CAD build for the part. Positions are in the model's coordinates, mm. Coordinates: 2 decimals unless noted, no trailing zeros. Loops run counter-clockwise (first coordinate to the right, second up) from the corner with the lowest first, then second, coordinate; pieces in that order, holes last. Notation, with made-up numbers: (74, -12.75) -> (122, -12.75) arc R20 ccw to (122, 9.25) -> close; hole circle Ø10 at (9, -33.75). An arc over 180 degrees is marked (long way). Write each question's results on one line, items separated by ' | '.
```python
from build123d import *

# Parameters (mm, degrees)
CROQUIS1_W              = 108
CROQUIS1_H              = 71
SALIENTE_EXTRUIR1_DEPTH = 1.5
CROQUIS2_W              = 8
CROQUIS2_H              = 3
CROQUIS2_W_2            = 12
CORTAR_EXTRUIR1_DEPTH   = 3
CROQUIS4_W              = 8
CROQUIS4_H              = 3
SALIENTE_EXTRUIR2_DEPTH = 3
REDONDEO1_R             = 4
CROQUIS5_R              = 1.5
CORTAR_EXTRUIR2_DEPTH   = 13
SIMETR_A2_START         = -1.5
SIMETR_A2_OUTLINE_R     = 1.5
SIMETR_A2_DEPTH         = 3
SIMETR_A2_2_DEPTH       = 3
CROQUIS6_W              = 3
CROQUIS6_H              = 14
CROQUIS6_H_2            = 8
CORTAR_EXTRUIR3_DEPTH   = 3
CROQUIS7_W              = 3.217414859
CROQUIS7_H              = 7.6
CORTAR_EXTRUIR4_DEPTH   = 73
CROQUIS10_W             = 12.8
CROQUIS10_H             = 9.989091156
CORTAR_EXTRUIR7_DEPTH   = 10
CROQUIS11_W             = 12.481361742
CROQUIS11_H             = 10
CORTAR_EXTRUIR8_DEPTH   = 10
CROQUIS12_R             = 2
CROQUIS12_R_2           = 3.661926667
CROQUIS12_R_3           = 5
CROQUIS12_W             = 4.5
CROQUIS12_H             = 7
CORTAR_EXTRUIR9_DEPTH   = 10
CORTAR_EXTRUIR10_DEPTH  = 10


# Read off the part's stored shape, not the designer's step: Simetría2
with BuildPart() as part:
    # Croquis1 → Saliente-Extruir1 (new, symmetric)
    with BuildSketch(Plane(origin=(0, 0, 0), x_dir=(0, 0, -1), z_dir=(1, 0, 0))):
        Rectangle(CROQUIS1_W, CROQUIS1_H)
    extrude(amount=SALIENTE_EXTRUIR1_DEPTH, both=True)

    # Croquis2 → Cortar-Extruir1 (cut)
    with BuildSketch(Plane.ZY.offset(1.5)):
        with Locations((-8, -34)):
            Rectangle(CROQUIS2_W, CROQUIS2_H)
        with Locations((8, -34)):
            Rectangle(CROQUIS2_W, CROQUIS2_H)
        with Locations((48, 34)):
            Rectangle(CROQUIS2_W_2, CROQUIS2_H)
        with Locations((24, 34)):
            Rectangle(CROQUIS2_W, CROQUIS2_H)
        with Locations((8, 34)):
            Rectangle(CROQUIS2_W, CROQUIS2_H)
        with Locations((-8, 34)):
            Rectangle(CROQUIS2_W, CROQUIS2_H)
        with Locations((-24, 34)):
            Rectangle(CROQUIS2_W, CROQUIS2_H)
        with Locations((-48, 34)):
            Rectangle(CROQUIS2_W_2, CROQUIS2_H)
    extrude(amount=-CORTAR_EXTRUIR1_DEPTH, mode=Mode.SUBTRACT)

    # Croquis4 → Saliente-Extruir2 (add)
    with BuildSketch(Plane.ZY.offset(1.5)):
        with Locations((16, 37)):
            Rectangle(CROQUIS4_W, CROQUIS4_H)
    extrude(amount=-SALIENTE_EXTRUIR2_DEPTH)

    # Redondeo1
    redondeo1_edges = [part.edges().sort_by_distance(p)[0] for p in [
        (0, 38.5, 20),
        (0, 38.5, 12),
    ]]
    fillet(redondeo1_edges, radius=REDONDEO1_R - 0.0001)  # a hair under: the kernel refuses the full size

    # Croquis5 → Cortar-Extruir2 (cut)
    with BuildSketch(Plane.ZY.offset(1.5)):
        with Locations((16, 33.5)):
            Circle(CROQUIS5_R)
    extrude(amount=-CORTAR_EXTRUIR2_DEPTH, mode=Mode.SUBTRACT)

    # Simetría2 outline → Simetría2 (cut)
    with BuildSketch(Plane.YZ.offset(SIMETR_A2_START)):
        with BuildLine():
            ThreePointArc((-34.5, 12), (-35.00401717, 12.031881215), (-35.5, 12.127016654))
            Line((-35.5, 12.127016654), (-35.5, 12))
            Line((-35.5, 12), (-34.5, 12))
        make_face()
        with Locations((-33.5, 16)):
            Circle(SIMETR_A2_OUTLINE_R)
    extrude(amount=SIMETR_A2_DEPTH, mode=Mode.SUBTRACT)

    # Simetr_a2 2 outline → Simetr_a2 2 (add)
    with BuildSketch(Plane.YZ.offset(SIMETR_A2_START)):
        with BuildLine():
            ThreePointArc((-35.5, 20), (-37.66227766, 18.576506397), (-38.5, 16.127016654))
            Line((-38.5, 16.127016654), (-38.5, 16))
            ThreePointArc((-38.5, 16), (-37.66227766, 13.550510257), (-35.5, 12.127016654))
            Line((-35.5, 12.127016654), (-35.5, 20))
        make_face()
    extrude(amount=SIMETR_A2_2_DEPTH)

    # Croquis6 → Cortar-Extruir3 (cut)
    with BuildSketch(Plane.ZY.offset(1.5)):
        with Locations((52.5, -28.5)):
            Rectangle(CROQUIS6_W, CROQUIS6_H)
        with Locations((52.5, -6.5)):
            Rectangle(CROQUIS6_W, CROQUIS6_H_2)
        with Locations((52.5, 6.5)):
            Rectangle(CROQUIS6_W, CROQUIS6_H_2)
        with Locations((52.5, 28.5)):
            Rectangle(CROQUIS6_W, CROQUIS6_H)
    extrude(amount=-CORTAR_EXTRUIR3_DEPTH, mode=Mode.SUBTRACT)

    # Croquis7 → Cortar-Extruir4 (cut)
    with BuildSketch(Plane(origin=(0, 32.5, 0), x_dir=(1, 0, 0), z_dir=(0, 1, 0))):
        with Locations((-0.10870743, 50.2)):
            Rectangle(CROQUIS7_W, CROQUIS7_H)
    extrude(amount=-CORTAR_EXTRUIR4_DEPTH, mode=Mode.SUBTRACT)

    # Croquis10 → Cortar-Extruir7 (cut)
    with BuildSketch(Plane.ZY.offset(1.5)):
        with Locations((-32.123797493, -27.505454422)):
            Rectangle(CROQUIS10_W, CROQUIS10_H)
    extrude(amount=-CORTAR_EXTRUIR7_DEPTH, mode=Mode.SUBTRACT)

    # Croquis11 → Cortar-Extruir8 (cut)
    with BuildSketch(Plane.ZY.offset(1.5)):
        with Locations((36.9, -27.5)):
            Rectangle(CROQUIS11_W, CROQUIS11_H)
    extrude(amount=-CORTAR_EXTRUIR8_DEPTH, mode=Mode.SUBTRACT)

    # Croquis12 → Cortar-Extruir9 (cut)
    with BuildSketch(Plane(origin=(1.5, 0, 0), x_dir=(0, 0, -1), z_dir=(1, 0, 0))):
        with Locations((4.6, -7.355454422)):
            Circle(CROQUIS12_R)
        with Locations((4.6, -24.855454422)):
            Circle(CROQUIS12_R)
        with Locations((14.4, -16.105454422)):
            Circle(CROQUIS12_R_2)
        with Locations((25.2, -16.105454422)):
            Circle(CROQUIS12_R_3)
        with Locations((-6.85, -16.105454422)):
            Rectangle(CROQUIS12_W, CROQUIS12_H)
    extrude(amount=-CORTAR_EXTRUIR9_DEPTH, mode=Mode.SUBTRACT)

    # Croquis13 → Cortar-Extruir10 (cut)
    with BuildSketch(Plane(origin=(1.5, 0, 0), x_dir=(0, 0, -1), z_dir=(1, 0, 0))):
        Polygon((46.4, 9.99), (46.4, 12.99), (42.65, 12.99), (42.65, 15.49), (39.65, 15.49), (39.65, 12.99), (38.4, 12.99), (38.4, 9.99), (39.65, 9.99), (39.65, 7.49), (42.65, 7.49), (42.65, 9.99), align=None)
    extrude(amount=-CORTAR_EXTRUIR10_DEPTH, mode=Mode.SUBTRACT)


solid = part.part
```
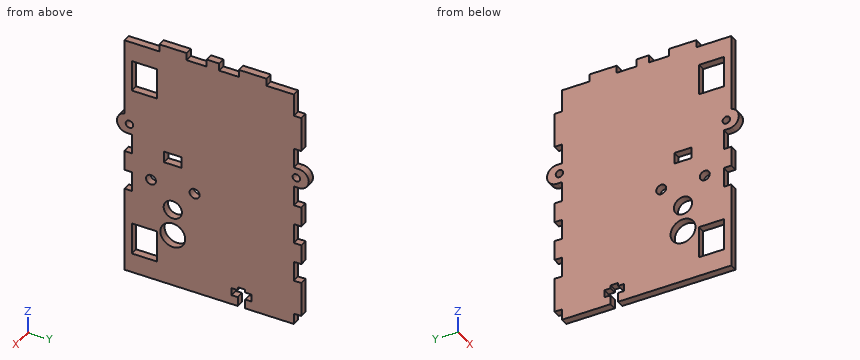
Q1. Cut at B-B on y = -14. Write the cut outline in (x, z), and give its area (3 significant figures).
Results are:
outline: (-1.5, -46.4) -> (1.5, -46.4) -> (1.5, -29.74) -> (-1.5, -29.74) -> close; (-1.5, -20.66) -> (1.5, -20.66) -> (1.5, -17.4) -> (-1.5, -17.4) -> close; (-1.5, -11.4) -> (1.5, -11.4) -> (1.5, 4.6) -> (-1.5, 4.6) -> close; (-1.5, 9.1) -> (1.5, 9.1) -> (1.5, 54) -> (-1.5, 54) -> close | area: 243 mm^2
Q2. Drop flat-ended pins along their axis: pin 1 (0.8 mm diameter, centred on x = -0.5, y = 9, fed in from +Z); pin 2 (0.9 mm diameter, centred on x = -0.5, z = 34, fed in from -Y). Give the stop position or say it passes through.
Results are:
pin 1: z = 51 | pin 2: y = -35.5
Q3. Cut at A-A on z = -21.5. Write the cut outline in (x, y).
Results are:
outline: (-1.5, -35.5) -> (1.5, -35.5) -> (1.5, -19.47) -> (-1.5, -19.47) -> close; (-1.5, -12.74) -> (1.5, -12.74) -> (1.5, 32.5) -> (-1.5, 32.5) -> close
Q4. Cut at C-C on x = -0.4. Give the number of separate pieces and of enclosed holes in the cut face, and give its area (3 significant figures).
Results are:
separate pieces: 1 | enclosed holes: 9 | area: 6,360 mm^2
Q5. Wall check: L1, parallel to Z at x = -0.55, y = -33.5; L2, parallel to Z at x = 1, y = -30; L3, parallel to Y at x = 1.05, z = -26. Give the ranges that are in metal, low to high. Write a range as from..to.
Results are:
L1: -46.4..-12, -4..4, 12..14.5, 17.5..51 | L2: -46.4..-38.52, -25.72..30.66, 43.14..51 | L3: -35.5..-32.5, -22.51..-21.04, -11.17..32.5
